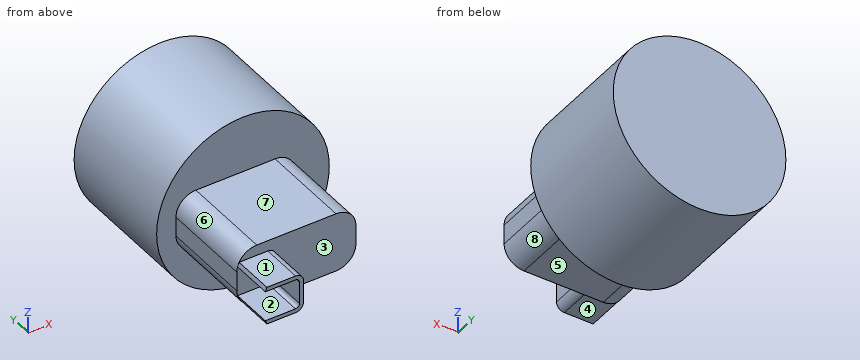
from build123d import *

# Parameters (mm, degrees)
SKETCH1_R           = 58
BOSS_EXTRUDE1_DEPTH = 83.82
BOSS_EXTRUDE2_DEPTH = 61.8
BOSS_EXTRUDE3_DEPTH = 90


with BuildPart() as part:
    # Sketch1 → Boss-Extrude1 (new body)
    with BuildSketch(Plane(origin=(0, 0, 0), x_dir=(1, 0, 0), z_dir=(0, 1, 0))):
        Circle(SKETCH1_R)
    extrude(amount=BOSS_EXTRUDE1_DEPTH)

    # Sketch2 → Boss-Extrude2 (add)
    with BuildSketch(Plane(origin=(0, 0, 0), x_dir=(1, 0, 0), z_dir=(0, 1, 0))):
        with BuildLine():
            Line((-45, -6.568854261), (-45, 6.568854261))
            ThreePointArc((-45, 6.568854261), (-41.075230868, 16.044085129), (-31.6, 19.968854261))
            Line((-31.6, 19.968854261), (21.6, 19.968854261))
            ThreePointArc((21.6, 19.968854261), (31.075230868, 16.044085129), (35, 6.568854261))
            Line((35, 6.568854261), (35, -6.568854261))
            ThreePointArc((35, -6.568854261), (31.075230868, -16.044085129), (21.6, -19.968854261))
            Line((21.6, -19.968854261), (-31.6, -19.968854261))
            ThreePointArc((-31.6, -19.968854261), (-41.075230868, -16.044085129), (-45, -6.568854261))
        make_face()
    extrude(amount=-BOSS_EXTRUDE2_DEPTH)

    # Sketch3 → Boss-Extrude3 (add)
    with BuildSketch(Plane(origin=(0, 0, 0), x_dir=(1, 0, 0), z_dir=(0, 1, 0))):
        with BuildLine():
            Line((-21.552493426, -4.8), (-21.552493426, 4.8))
            Line((-21.552493426, 4.8), (-21.552493426, 7.4))
            ThreePointArc((-21.552493426, 7.4), (-22.343305117, 9.309188309), (-24.252493426, 10.1))
            Line((-24.252493426, 10.1), (-26.852493426, 10.1))
            Line((-26.852493426, 10.1), (-44.526368777, 10.1))
            Line((-44.526368777, 10.1), (-43.463086562, 12.8))
            Line((-43.463086562, 12.8), (-24.152493426, 12.8))
            ThreePointArc((-24.152493426, 12.8), (-20.404827486, 11.24766594), (-18.852493426, 7.5))
            Line((-18.852493426, 7.5), (-18.852493426, -7.5))
            ThreePointArc((-18.852493426, -7.5), (-20.404827486, -11.24766594), (-24.152493426, -12.8))
            Line((-24.152493426, -12.8), (-40.189232196, -12.8))
            Line((-40.189232196, -12.8), (-43.463086562, -12.8))
            Line((-43.463086562, -12.8), (-44.526368777, -10.1))
            Line((-44.526368777, -10.1), (-26.852493426, -10.1))
            Line((-26.852493426, -10.1), (-24.252493426, -10.1))
            ThreePointArc((-24.252493426, -10.1), (-22.343305117, -9.309188309), (-21.552493426, -7.4))
            Line((-21.552493426, -7.4), (-21.552493426, -4.8))
        make_face()
    extrude(amount=-BOSS_EXTRUDE3_DEPTH)


solid = part.part
Geometry: final body of the model. Coordinates: model frame, mm. Face numbers are marked on the shaded views. A direction names the side the tool comes from. Round coordinates to 2 decimals unless told otherwise and drop trailing zeros. Loops run counter-clockwise (first coordinate to the right, second up) from the corner with the lowest first, then second, coordinate; pieces in that order, holes last. Notation, with made-up numbers: M -33,10 L -14,10 A27 ccw -14,48 Z; hole C 15,19 d9. An arc over 180 degrees is marked long. One line per question, with ' | ' between items.
(1) Cut plane C-C on x = 0. Return the cut outline in (y, z), plus the area to 3 significant figures.
Check result:
outline: M -61.8,-19.97 L 0,-19.97 L 0,-58 L 83.82,-58 L 83.82,58 L 0,58 L 0,19.97 L -61.8,19.97 Z | area: 12,200 mm2
(2) Material intervals for line 1 along Y through (x, z) = (45.5, -1); line 2 along Y through (x, z) = (26, 1); line 3 along X through (y, z) = (10.5, -2), sorted ascending. Write a range as from..to.
Check result:
line 1: y = 0..83.82 | line 2: y = -61.8..83.82 | line 3: x = -57.97..57.97
(3) Cut plane B-B on z = 0. Return the cut outline in (x, y).
Check result:
outline: M -58,0 L -45,0 L -45,-61.8 L -21.55,-61.8 L -21.55,-90 L -18.85,-90 L -18.85,-61.8 L 35,-61.8 L 35,0 L 58,0 L 58,83.82 L -58,83.82 Z
(4) Contact query for flat-ended pins moving along their axis: P1, Ø7.5, axis at y = -82, z = -1, coming from the -X side; P2, Ø4, axis at x = -27.5, y = -46, coming from the -Z side; P3, Ø9.5, axis at x = -38, y = -79, coming from the +Z side. Output: stop coordinate, or through.
Check result:
P1: stops at x = -21.55 | P2: stops at z = -19.97 | P3: stops at z = 12.8
(5) Pull-direction query (Z, two-part tool) for the marked faces 1, 2, 3 and 4; classes: +Z half, -Z half, draft (parallel to the pull), parting line (faces both ways), or undercut.
Check result:
face 1: +Z half | face 2: undercut | face 3: draft | face 4: -Z half
(6) Access query for the marked faces 5, 6, 7 and 8. Directions: +Z, -Z, +X, -X, +Y, -Y. A direction counts if a zero-diameter tool reaches every point of the face in a straight line with its end or side. Return the directions, or none.
Check result:
face 5: -Z, +X, -X, -Y | face 6: +Z, -X, -Y | face 7: +Z, +X, -X, -Y | face 8: -Z, +X, -Y
(7) Cut plane A-A on y = -54. Return the cut outline in (x, z), plus the area to 3 significant figures.
Check result:
outline: M -45,-6.57 A13.4 ccw -31.6,-19.97 L 21.6,-19.97 A13.4 ccw 35,-6.57 L 35,6.57 A13.4 ccw 21.6,19.97 L -31.6,19.97 A13.4 ccw -45,6.57 Z | area: 3,040 mm2
(8) Cut plane D-D on y = 9. Return the cut outline in (x, z), plus the area to 3 significant figures.
Check result:
outline: C 0,0 d116 | area: 10,600 mm2
